Check sheet for the modelled part. Datum: model origin and axes. Units: mm. Face numbers are marked on the shaded views. Round coordinates to 2 decimals unless told otherwise and drop trailing zeros. Write each loop counter-clockwise with the first axis right and the second up, starting at its lowest first coordinate (ties: lowest second). Pieces come first, ordered by that corner, then holes. Notation, with made-up numbers: (19.25, 25.5) -> (45.25, 25.5) arc R32 ccw to (45.25, 63.5) -> close; hole circle Ø1 at (10.25, 83.25). An arc over 180 degrees is marked (long way). Write item = value, one per line.
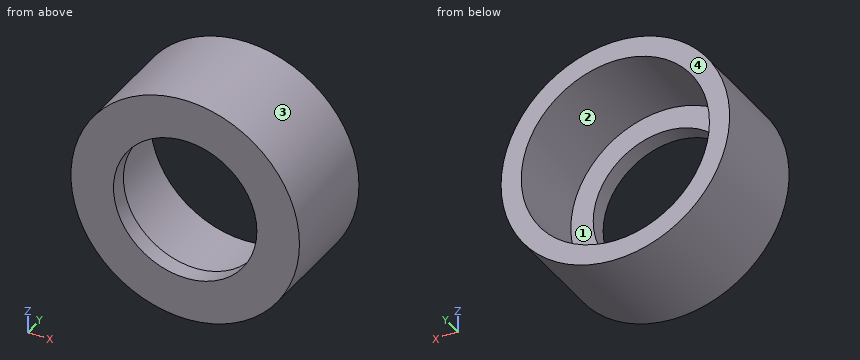
from build123d import *

# Parameters (mm, degrees)
SKETCH019_R   = 16.66875
PAD019_DEPTH  = 15.875
SKETCH018_R   = 20.240625
SKETCH018_R_2 = 12.7
PAD018_DEPTH  = 19.05


with BuildPart() as body019:
    # Sketch019 → Pad019 (new body)
    with BuildSketch(Plane.XZ):
        Circle(SKETCH019_R)
    extrude(amount=PAD019_DEPTH)


with BuildPart() as cut012:
    # Sketch018 → Pad018 (new body)
    with BuildSketch(Plane.XZ):
        Circle(SKETCH018_R)
        Circle(SKETCH018_R_2, mode=Mode.SUBTRACT)
    extrude(amount=PAD018_DEPTH)

    # Cut012: cut Body019
    add(body019.part, mode=Mode.SUBTRACT)


with BuildPart() as cut012_1:
    # Cut012 placement: moved
    add(cut012.part.moved(Location((0, -29.37, 0))))


solid = cut012_1.part
(1) Sectioned sample at C-C on y = -32.25. Enter the section's corners in (x, z).
Worked answers:
outline = circle Ø40.48 at (0, 0); hole circle Ø33.34 at (0, 0)
(2) Release check for a two-part mould opening along Z. For the marked faces 1, 2, 3 and 4 record: pulls with the +Z half, pulls with the -Z half, needs draft (parallel to the pull), parting line crosses it, or undercut.
Worked answers:
face_1 = undercut
face_2 = undercut
face_3 = parting line crosses it
face_4 = needs draft
(3) Sectioned sample at A-A on x = 0. Enter the section's corners in (y, z) (3 decimals), then the cut area to 3 significant figures.
Worked answers:
outline = (-48.42, -20.241) -> (-29.37, -20.241) -> (-29.37, -16.669) -> (-45.245, -16.669) -> (-45.245, -12.7) -> (-48.42, -12.7) -> close; (-48.42, 12.7) -> (-45.245, 12.7) -> (-45.245, 16.669) -> (-29.37, 16.669) -> (-29.37, 20.241) -> (-48.42, 20.241) -> close
area = 161 mm²
(4) Sectioned sample at B-B on z = 0. Enter the section's corners in (x, y) (3 decimals).
Worked answers:
outline = (-20.241, -48.42) -> (-12.7, -48.42) -> (-12.7, -45.245) -> (-16.669, -45.245) -> (-16.669, -29.37) -> (-20.241, -29.37) -> close; (12.7, -48.42) -> (20.241, -48.42) -> (20.241, -29.37) -> (16.669, -29.37) -> (16.669, -45.245) -> (12.7, -45.245) -> close
(5) Go/stop test with flat-tipped pins: P1, Ø2, axis at x = 2, y = -41.5, coming from the -Z side; P2, Ø5, axis at y = -37.5, z = 6.5, coming from the -X side; P3, Ø3, axis at x = -13, y = -43.5, coming from the +Z side; P4, Ø1.5, axis at x = 10.5, z = 3, coming from the -Y side. Record where each tip stops, or that it passes through.
Worked answers:
P1 = -20.22
P2 = -19.84
P3 = 16.66
P4 = through
(6) Material ranges on L1, parallel to Z at x = 0, y = -46.5; L2, parallel to Z at x = 0, y = -34.5; L3, parallel to Y at x = 12.5, z = 10.5 (3 decimals), recorded low to high. Write a range as [from, to].
Worked answers:
L1 = [-20.24, -12.7], [12.7, 20.24]
L2 = [-20.24, -16.67], [16.67, 20.24]
L3 = [-48.42, -45.245]
